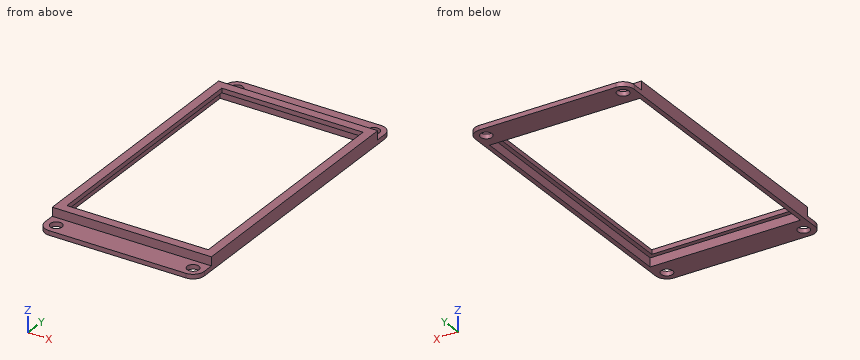
from build123d import *

# Parameters (mm, degrees)
F0_W     = 56.515
F0_H     = 92.075
F0_W_2   = 53.34
F0_H_2   = 88.9
F1_DEPTH = 1.524
F2_W     = 56.515
F2_H     = 107.95
F2_R     = 2.0828
F2_W_2   = 53.34
F2_H_2   = 88.9
F3_DEPTH = 1.5875
F4_W     = 56.515
F4_H     = 92.075
F4_W_2   = 50.165
F4_H_2   = 85.725
F5_DEPTH = 1.5875
F6_R     = 3.96875


with BuildPart() as f1:
    # F0 (on Top) → F1 (new body)
    with BuildSketch(Plane.XY):
        Rectangle(F0_W, F0_H)
        Rectangle(F0_W_2, F0_H_2, mode=Mode.SUBTRACT)
    extrude(amount=F1_DEPTH)

    # F2 (on face) → F3 (join)
    with BuildSketch(Plane(origin=(0, 0, 0), x_dir=(1, 0, 0), z_dir=(0, 0, -1))):
        Rectangle(F2_W, F2_H)
        with Locations((-24.28875, -50.00625)):
            Circle(F2_R, mode=Mode.SUBTRACT)
        with Locations((24.28875, -50.00625)):
            Circle(F2_R, mode=Mode.SUBTRACT)
        with Locations((-24.28875, 50.00625)):
            Circle(F2_R, mode=Mode.SUBTRACT)
        Rectangle(F2_W_2, F2_H_2, mode=Mode.SUBTRACT)
        with Locations((24.28875, 50.00625)):
            Circle(F2_R, mode=Mode.SUBTRACT)
    extrude(amount=F3_DEPTH)

    # F4 (on face) → F5 (join)
    with BuildSketch(Plane.XY.offset(1.524)):
        Rectangle(F4_W, F4_H)
        Rectangle(F4_W_2, F4_H_2, mode=Mode.SUBTRACT)
    extrude(amount=F5_DEPTH)

    # F6
    f6_edges = [f1.edges().sort_by_distance(p)[0] for p in [
        (-28.2575, -53.975, -0.79375),
        (28.2575, -53.975, -0.79375),
        (28.2575, 53.975, -0.79375),
        (-28.2575, 53.975, -0.79375),
    ]]
    fillet(f6_edges, radius=F6_R)


solid = f1.part
Could you check a few things on this model? Use its own coordinates, in mm. Give positions to 0.01 mm unless a question says otherwise; leave off trailing zeros. Order: outer loops, then holes, each group sorted by start corner. A loop starts at its lowest first (then second) coordinate and runs counter-clockwise, first axis right, second up. Notation, with made-up numbers: (86, -20.75) - (92, -20.75) arc R19 ccw to (92, 1.25) - close; hole circle Ø10 at (-2.75, -25.75). An arc over 180 degrees is marked (long way). One line per item, written item: value. Start each with the question number.
1. Imagine slicing it at B-B on y = 9. List the corners of the cut face in (x, z) for me, plus the area to 3 significant figures.
2. If I drill on probe 1 along Y at (x, z) = (-13, 0.15); probe 2 along X at (y, z) = (-21, -1); probe 3 along Y at (x, z) = (-14, -1.05) (3 decimals), over which ranges is the centre line in solid material (lowest first)?
3. For P1, Ø0.9, axis at x = 4.5, z = 2, coming from the +Y side; P2, Ø2.5, axis at x = 13, y = -51, coming from the +Z side; P3, Ø5, axis at x = 24.29, y = 50.01, coming from the -Z side; P4, Ø2.5, axis at x = -24.29, y = -50.01, coming from the -Z side, each with a flat end and sliding along its axis, tell me the tip position at first contact or that it passes through.
Values:
1. outline: (-28.26, -1.59) - (-26.67, -1.59) - (-26.67, 1.52) - (-25.08, 1.52) - (-25.08, 3.11) - (-28.26, 3.11) - close; (25.08, 1.52) - (26.67, 1.52) - (26.67, -1.59) - (28.26, -1.59) - (28.26, 3.11) - (25.08, 3.11) - close
1. area: 20.0 mm²
2. probe 1: -46.04 to -44.45, 44.45 to 46.04
2. probe 2: -28.26 to -26.67, 26.67 to 28.26
2. probe 3: -53.975 to -44.45, 44.45 to 53.975
3. P1: y = 46.04
3. P2: z = 0
3. P3: z = -1.59
3. P4: through
